Source: three-view drawing plus pictorial views. Frame: mm from the lowest corner of the part. A direction names the side the tool comes from. Give positions to 0.01 mm unless a question says otherwise; leave off trailing zeros. Write each loop counter-clockwise with the first axis right and the second up, starting at its lowest first coordinate (ties: lowest second). Pieces come first, ordered by that corner, then holes.
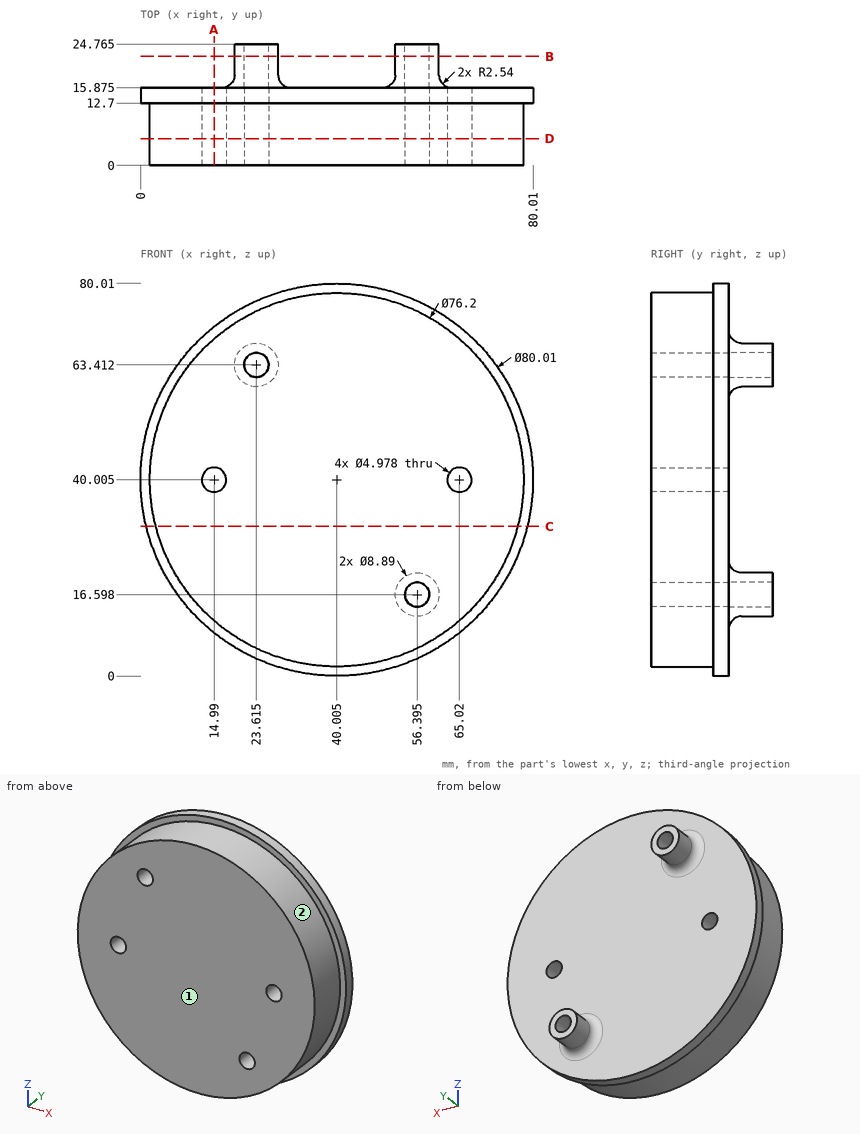
Q1. Ray query, line 1 along X through (y, z) = (5.5, 39); line 2 along Y through (x, z) = (22.5, 23.5) (1 decimal); line 3 along X through (y, z) = (7, 14.5) (1 decimal). Return the intervals inside material, ascending.
Filled sheet:
line 1: x = 1.92 to 12.71, 17.27 to 62.74, 67.3 to 78.09
line 2: y = 0 to 15.9
line 3: x = 11.7 to 55.1, 57.7 to 68.3
Q2. Section A-A on x = 14.99. Output: boundary loops of the cut face in (y, z) (1 decimal), plus the area to 3 significant figures.
Filled sheet:
outline: (0, 11.3) - (12.7, 11.3) - (12.7, 8.8) - (15.9, 8.8) - (15.9, 37.5) - (0, 37.5) - close; (0, 42.5) - (15.9, 42.5) - (15.9, 71.2) - (12.7, 71.2) - (12.7, 68.7) - (0, 68.7) - close
area: 849 mm2
Q3. Section C-C on z = 30.5. Output: boundary loops of the cut face in (x, y) (1 decimal).
Filled sheet:
outline: (1.1, 12.7) - (3.1, 12.7) - (3.1, 0) - (76.9, 0) - (76.9, 12.7) - (78.9, 12.7) - (78.9, 15.9) - (1.1, 15.9) - close
Q4. Access query for the marked faces 1 and 2. Directions: +Z, -Z, +X, -X, +Y, -Y. A direction counts if a zero-diameter tool reaches every point of the face in a straight line with its end or side. Return the directions, or none.
Filled sheet:
face 1: +Z, -Z, +X, -X, -Y
face 2: -Y
Q5. Pin query (flat end, axial travel): P1, Ø2, axis at x = 9, y = 6, coming from the +Z side (1 decimal); P2, Ø4.5, axis at x = 65.02, z = 40.005, coming from the +Y side; P3, Ø6, axis at x = 10.5, z = 20, coming from the +Y side (3 decimals); P4, Ø1.5, axis at x = 44.5, y = 7, coming from the +Z side. Return the tip coordinate at first contact, or that it passes through.
Filled sheet:
P1: stops at z = 63.5
P2: passes through
P3: stops at y = 15.875
P4: stops at z = 77.92
Q6. Section D-D on y = 5.5. Output: boundary loops of the cut face in (x, z) (1 decimal), plus the area to 3 significant figures.
Filled sheet:
outline: circle Ø76.2 at (40, 40); hole circle Ø5 at (15, 40); hole circle Ø5 at (23.6, 63.4); hole circle Ø5 at (56.4, 16.6); hole circle Ø5 at (65, 40)
area: 4,480 mm2
Q7. Section B-B on y = 22.25. Output: boundary loops of the cut face in (x, z) (1 decimal).
Filled sheet:
outline: circle Ø8.9 at (23.6, 63.4); circle Ø8.9 at (56.4, 16.6); hole circle Ø5 at (23.6, 63.4); hole circle Ø5 at (56.4, 16.6)
